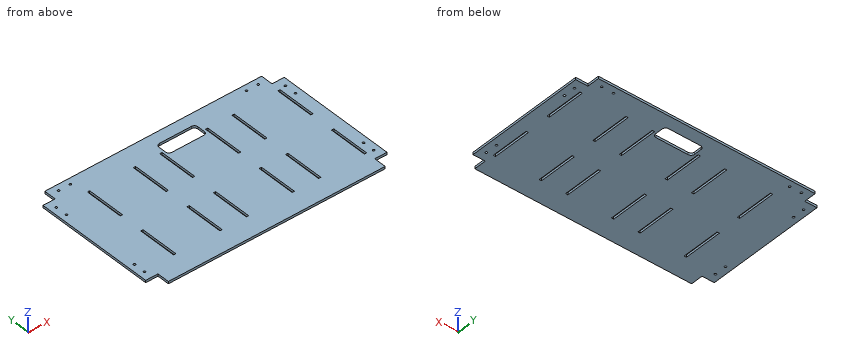
from build123d import *

# Parameters (mm, degrees)
SKETCH_1_W          = 500.8
SKETCH_1_H          = 300.8
EXTRUDE_1_DEPTH     = 4.75
SKETCH_2_W          = 25.4
SKETCH_2_H          = 25.4
SKETCH_2_W_2        = 4.75
SKETCH_2_H_2        = 80
CUT_EXTRUDE_1_DEPTH = 10
SKETCH_3_R          = 2.150000004
SKETCH_3_R_2        = 2.15
CUT_EXTRUDE_2_DEPTH = 5
SKETCH_4_W          = 80.5
SKETCH_4_H          = 30
CUT_EXTRUDE_3_DEPTH = 4.75
FILLET_1_R          = 7


with BuildPart() as part:
    # 草圖1 → 填料-伸長1 (new body)
    with BuildSketch(Plane.XY):
        Rectangle(SKETCH_1_W, SKETCH_1_H)
    extrude(amount=EXTRUDE_1_DEPTH)

    # 草圖2 → 除料-伸長1 (cut)
    with BuildSketch(Plane(origin=(0, 0, 0), x_dir=(-1, 0, 0), z_dir=(0, 0, -1))):
        with Locations((-237.7, 137.7)):
            Rectangle(SKETCH_2_W, SKETCH_2_H)
        with Locations((-237.7, -137.7)):
            Rectangle(SKETCH_2_W, SKETCH_2_H)
        with Locations((237.7, 137.7)):
            Rectangle(SKETCH_2_W, SKETCH_2_H)
        with Locations((237.7, -137.7)):
            Rectangle(SKETCH_2_W, SKETCH_2_H)
        with Locations((-222.625, 65.4)):
            Rectangle(SKETCH_2_W_2, SKETCH_2_H_2)
        with Locations((-222.625, -65.4)):
            Rectangle(SKETCH_2_W_2, SKETCH_2_H_2)
        with Locations((172.625, 65.4)):
            Rectangle(SKETCH_2_W_2, SKETCH_2_H_2)
        with Locations((172.625, -64.4)):
            Rectangle(SKETCH_2_W_2, SKETCH_2_H_2)
        with Locations((-127.375, 65.4)):
            Rectangle(SKETCH_2_W_2, SKETCH_2_H_2)
        with Locations((-72.625, 65.4)):
            Rectangle(SKETCH_2_W_2, SKETCH_2_H_2)
        with Locations((22.625, 65.4)):
            Rectangle(SKETCH_2_W_2, SKETCH_2_H_2)
        with Locations((77.375, 65.4)):
            Rectangle(SKETCH_2_W_2, SKETCH_2_H_2)
        with Locations((77.375, -65.4)):
            Rectangle(SKETCH_2_W_2, SKETCH_2_H_2)
        with Locations((22.625, -65.4)):
            Rectangle(SKETCH_2_W_2, SKETCH_2_H_2)
        with Locations((-127.375, -65.4)):
            Rectangle(SKETCH_2_W_2, SKETCH_2_H_2)
        with Locations((-72.625, -65.4)):
            Rectangle(SKETCH_2_W_2, SKETCH_2_H_2)
    extrude(amount=-CUT_EXTRUDE_1_DEPTH, mode=Mode.SUBTRACT)

    # 草圖3 → 除料-伸長2 (cut)
    with BuildSketch(Plane.XY.offset(4.75)):
        with Locations((-237.7, 107.300000013)):
            Circle(SKETCH_3_R)
        with Locations((-237.7, 82.800000013)):
            Circle(SKETCH_3_R)
        with Locations((-207.3, 137.700000006)):
            Circle(SKETCH_3_R_2)
        with Locations((-182.8, 137.700000006)):
            Circle(SKETCH_3_R_2)
        with Locations((-237.7, -82.800000001)):
            Circle(SKETCH_3_R_2)
        with Locations((-237.7, -107.300000001)):
            Circle(SKETCH_3_R_2)
        with Locations((237.7, -107.300000007)):
            Circle(SKETCH_3_R)
        with Locations((237.7, -82.800000007)):
            Circle(SKETCH_3_R)
        with Locations((237.7, 107.300000006)):
            Circle(SKETCH_3_R_2)
        with Locations((237.7, 82.800000006)):
            Circle(SKETCH_3_R_2)
        with Locations((182.8, 137.700000006)):
            Circle(SKETCH_3_R_2)
        with Locations((207.3, 137.700000006)):
            Circle(SKETCH_3_R_2)
    extrude(amount=-CUT_EXTRUDE_2_DEPTH, mode=Mode.SUBTRACT)

    # 草圖4 → 除料-伸長3 (cut)
    with BuildSketch(Plane.XY.offset(4.75)):
        with Locations((25, 110.4)):
            Rectangle(SKETCH_4_W, SKETCH_4_H)
    extrude(amount=-CUT_EXTRUDE_3_DEPTH, mode=Mode.SUBTRACT)

    # 圓角1
    fillet_1_edges = [part.edges().sort_by_distance(p)[0] for p in [
        (65.25, 125.4, 2.375),
        (65.25, 95.4, 2.375),
        (-15.25, 95.4, 2.375),
        (-15.25, 125.4, 2.375),
    ]]
    fillet(fillet_1_edges, radius=FILLET_1_R)


solid = part.part
Read the model definition and answer for the solid it produces. Units are mm, in the model's axes. Give positions to 0.01 mm unless a question says otherwise; leave off trailing zeros. Loops run counter-clockwise (first coordinate to the right, second up) from the corner with the lowest first, then second, coordinate; pieces in that order, holes last. Notation, with made-up numbers: (72, 78.5) - (101, 78.5) arc R21 ccw to (101, 95.5) - close; hole circle Ø1 at (34, -23). An arc over 180 degrees is marked (long way). Answer as CSV lines item,"result". Start each with the question number.
1) Find section A-A (y = -90.5). Write down the section's boundary in (x, z), then the cut area to 3 significant figures.
2) Find section B-B (z = 0.85). State how many separate pieces and enclosed holes the cut face has, then the cut area to 3 significant figures.
3) Each of these flat-tipped pins is pushed along its axis until it touches: pin 1 Ø1.4 at (y, z) = (135.5, 2.5) entering from +X; pin 2 Ø1.4 at (x, z) = (238.5, 3) entering from +Y; pin 3 Ø1.4 at (y, z) = (138.5, 2) entering from -X. Where does it stop, or does it pass through?
4) Straight lines are drawn through the part: L1, parallel to Y at x = -237.7, z = 2.65; L2, parallel to X at y = -107.3, z = 1.7; L3, parallel to Y at x = -182.8, z = 1.3. For each, find the intervals that lie inside material, in ascending order. Write a range as from..to.
Findings below:
1,outline,"(-250.4, 0) - (-175, 0) - (-175, 4.75) - (-250.4, 4.75) - close; (-170.25, 0) - (-79.75, 0) - (-79.75, 4.75) - (-170.25, 4.75) - close; (-75, 0) - (-25, 0) - (-25, 4.75) - (-75, 4.75) - close; (-20.25, 0) - (70.25, 0) - (70.25, 4.75) - (-20.25, 4.75) - close; (75, 0) - (125, 0) - (125, 4.75) - (75, 4.75) - close; (129.75, 0) - (220.25, 0) - (220.25, 4.75) - (129.75, 4.75) - close; (225, 0) - (250.4, 0) - (250.4, 4.75) - (225, 4.75) - close"
1,area,"2,240 mm^2"
2,separate pieces,"1"
2,enclosed holes,"25"
2,area,"141,000 mm^2"
3,pin 1,"x = 225"
3,pin 2,"y = 125"
3,pin 3,"x = -225"
4,L1,"-125..-109.45, -105.15..-84.95, -80.65..80.65, 84.95..105.15, 109.45..125"
4,L2,"-250.4..-239.85, -235.55..235.55, 239.85..250.4"
4,L3,"-150.4..135.55, 139.85..150.4"
